Part model, mm, in its own coordinate system. Give positions to 0.01 mm unless a question says otherwise; leave off trailing zeros. Write each loop counter-clockwise with the first axis right and the second up, starting at its lowest first coordinate (ties: lowest second). Pieces come first, ordered by that corner, then holes. Notation, with made-up numbers: (-17.75, 7) - (9.25, 7) arc R22 ccw to (9.25, 35) - close; hole circle Ø2 at (80, 37.5). An arc over 180 degrees is marked (long way). Answer in a Markdown table with one row per item. Add a question column.
1. Band-saw the part on D-D on x = -7.5. Write the cut outline in (y, z).
2. Drop flat-ended pins along their axis: pin 1 Ø1.5 at (x, y) = (28, 2) entering from -Z; pin 2 Ø2 at (y, z) = (2.5, -28) entering from -X; pin 3 Ø1.5 at (y, z) = (3, 11.5) entering from -X. Give the stop position or say it passes through.
3. Probe line 1 along X through (y, z) = (1.05, 6.5); line 2 along X through (y, z) = (0.8, 3.5); line 3 along Z through (x, y) = (-10.5, 4). List the from-to ranges inside material, lowest first.
4. Band-saw the part on A-A on z = -26. Write the cut outline in (x, y), plus the area to 3 significant figures.
5. Band-saw the part on C-C on z = 7.5. Write the cut outline in (x, y), plus the area to 3 significant figures.
6. Band-saw the part on B-B on y = 2.1. Write the cut outline in (x, z).
Solid Edge part; units mm, degrees
sketch "Sketch1" plane through (0, 0, 0) normal (0, -1, 0) x (1, 0, 0)
  arc A0 (-50, -15) -> (-10, 25) centre (-10, -15) cw
  line L0 (-2.5, 25) -> (-10, 25)
  line L1 (-2.5, 0) -> (-2.5, 25)
  line L2 (2.5, 0) -> (-2.5, 0)
  line L3 (2.5, 25) -> (2.5, 0)
  line L4 (10, 25) -> (2.5, 25)
  arc A1 (10, 25) -> (50, -15) centre (10, -15) cw
  line L5 (50, -25) -> (50, -15)
  line L6 (32.5, -25) -> (50, -25)
  line L7 (32.5, -29.067) -> (32.5, -25)
  line L8 (17.5, -29.067) -> (32.5, -29.067)
  line L9 (17.5, -25) -> (17.5, -29.067)
  line L10 (-17.5, -25) -> (17.5, -25)
  line L11 (-17.5, -29.6011) -> (-17.5, -25)
  line L12 (-32.5, -29.6011) -> (-17.5, -29.6011)
  line L13 (-32.5, -25) -> (-32.5, -29.6011)
  line L14 (-50, -25) -> (-32.5, -25)
  line L15 (-50, -15) -> (-50, -25)
extrude "Protrusion1" add sketch "Sketch1" against normal blind 5
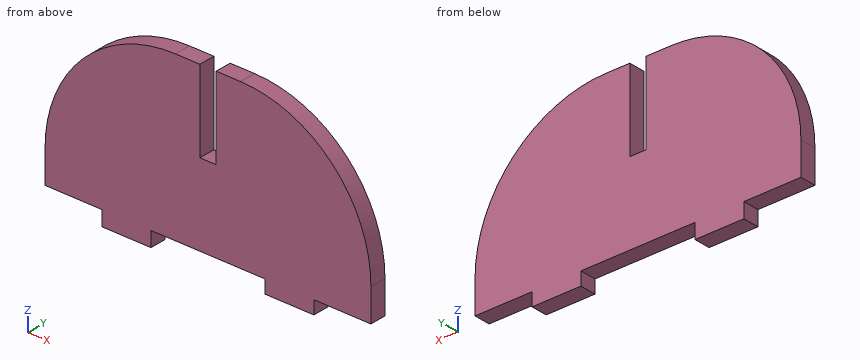
Values:
| question | item | result |
|---|---|---|
| 1 | outline | (0, -25) - (5, -25) - (5, 25) - (0, 25) - close |
| 2 | pin 1 | stops at z = -29.07 |
| 2 | pin 2 | stops at x = -32.5 |
| 2 | pin 3 | stops at x = -40.61 |
| 3 | line 1 | x = -43.73 to -2.5, 2.5 to 43.73 |
| 3 | line 2 | x = -45.46 to -2.5, 2.5 to 45.46 |
| 3 | line 3 | z = -25 to 25 |
| 4 | outline | (-32.5, 0) - (-17.5, 0) - (-17.5, 5) - (-32.5, 5) - close; (17.5, 0) - (32.5, 0) - (32.5, 5) - (17.5, 5) - close |
| 4 | area | 150 mm² |
| 5 | outline | (-43.07, 0) - (-2.5, 0) - (-2.5, 5) - (-43.07, 5) - close; (2.5, 0) - (43.07, 0) - (43.07, 5) - (2.5, 5) - close |
| 5 | area | 406 mm² |
| 6 | outline | (-50, -25) - (-32.5, -25) - (-32.5, -29.6) - (-17.5, -29.6) - (-17.5, -25) - (17.5, -25) - (17.5, -29.07) - (32.5, -29.07) - (32.5, -25) - (50, -25) - (50, -15) arc R40 ccw to (10, 25) - (2.5, 25) - (2.5, 0) - (-2.5, 0) - (-2.5, 25) - (-10, 25) arc R40 ccw to (-50, -15) - close |
